Verification items for the finished model (mm, model axes). A direction names the side the tool comes from. Round coordinates to 2 decimals unless told otherwise and drop trailing zeros. Write each loop counter-clockwise with the first axis right and the second up, starting at its lowest first coordinate (ties: lowest second). Pieces come first, ordered by that corner, then holes. Notation, with made-up numbers: (81, 39) - (94, 39) arc R9 ccw to (94, 55) - close; hole circle Ø2 at (61, 17.5). An arc over 180 degrees is marked (long way). Answer as a JSON object with one key per item and string values. Group by question number.
1) Set-up check for faces 1 (the cylindrical face through (-13.753, 5.143, -125.535)), 2 (the flat face through (-72, 10, -123)), 3 (the flat face through (-72, 5, -128)), 4 (the flat face through (-95, 15, -128)): record each of +Z, -Z, +X, -X, +Y, -Y from which the full face is reachable in a straight line by a thin tool's end or side.
2) Mould release check, pull along X, two halves, no side actions. Record for faces 5 (the flat face through (-95, 10, -148)), 6 (the flat face through (-44, 14.9, -120.7)), 7 (the flat face through (-90, 14.9, -170.7)): +X half, -X half, draft (parallel to the pull), parting line (faces both ways), or undercut.
3) Section check D-D (x = -82). Enter the section's corners in (y, z).
4) Section check C-C (z = -16). Enter the section's corners in (x, y).
5) Thickness scan on line 1 (Z direction, x = -81.5, y = 8.75); line 2 (Z direction, x = -67, y = 3.25); line 3 (X direction, y = 8.2, z = -31). Record the ranges inside material, lowest first.
6) Section check B-B (z = -154). Enter the section's corners in (x, y).
7) Section check A-A (x = -5). Enter the section's corners in (y, z).
8) Go/stop test with flat-tipped pins: pin 1 Ø3 at (x, z) = (-27.5, -122.5) entering from +Y; pin 2 Ø11 at (x, y) = (-19.5, 4) entering from -Z; pin 3 Ø11 at (x, y) = (-50.5, 17.5) entering from +Z. Record where each tip stops, or that it passes through.
Autodesk Inventor part; units mm, degrees
ref_plane "YZ Plane" through (0, 0, 0) normal (1, 0, 0) x (0, 1, 0)
ref_plane "XZ Plane" through (0, 0, 0) normal (0, 1, 0) x (-1, 0, 0)
ref_plane "XY Plane" through (0, 0, 0) normal (0, 0, 1) x (1, 0, 0)
sketch "Sketch1" plane through (0, 0, 0) normal (0, 1, 0) x (-1, 0, 0)
  line L0 (0, 0) -> (100, 0)
  line L1 (100, 0) -> (100, -178)
  line L2 (0, -178) -> (0, 0)
  line L3 (90, -10) -> (10, -10)
  line L4 (90, -52) -> (10, -52)
  line L5 (90, -62) -> (10, -62)
  line L6 (90, -52) -> (90, -10)
  line L7 (10, -10) -> (10, -52)
  line L8 (90, -118) -> (10, -118)
  line L9 (90, -168) -> (90, -128)
  line L10 (90, -118) -> (90, -62)
  line L11 (10, -62) -> (10, -118)
  line L12 (10, -128) -> (10, -168)
  line L13 (100, -178) -> (90, -178)
  line L14 (10, -178) -> (0, -178)
  line L15 (90, -168) -> (90, -178)
  line L16 (10, -168) -> (44, -168)
  line L17 (54, -168) -> (54, -178)
  line L18 (54, -178) -> (10, -178)
  line L19 (54, -168) -> (54, -128)
  line L20 (44, -128) -> (44, -168)
  line L21 (90, -128) -> (54, -128)
  line L22 (44, -128) -> (10, -128)
  dimension "thickness" = 10
  dimension "d3" = 10
  dimension "d4" = 10
  dimension "d8" = 10
  dimension "motor" = 42
  dimension "d10" = 10
  dimension "d11" = 10
  dimension "d27" = 10
  dimension "batterywidth" = 56
  dimension "d31" = 80
  dimension "suspensionWidth" = 40
  dimension "d33" = 10
  dimension "d34" = 10
  dimension "d36" = 10
  dimension "d38" = 10
  dimension "d39" = 40
  dimension "d40" = 40
  dimension "d41" = 34
  dimension "d215" = 36
extrude "Extrusion2" add sketch "Sketch1" along normal blind 10
sketch "Sketch2" plane through (0, 10, 0) normal (0, 1, 0) x (1, 0, 0)
  line L0 (-100, 0) -> (-90, 0)
  line L1 (-90, 0) -> (-90, 10)
  line L2 (-90, 10) -> (-100, 10)
  line L3 (-100, 10) -> (-100, 0)
  line L4 (-10, 52) -> (-10, 10)
  line L5 (0, 0) -> (-10, 0)
  line L6 (-10, 0) -> (-10, 10)
  line L7 (-10, 10) -> (0, 10)
  line L8 (0, 10) -> (0, 0)
  line L9 (-100, 178) -> (-100, 0)
  line L10 (-100, 0) -> (0, 0)
  line L11 (-100, 52) -> (-90, 52)
  line L12 (-90, 52) -> (-90, 62)
  line L13 (-90, 62) -> (-100, 62)
  line L14 (-100, 62) -> (-100, 52)
  line L15 (-90, 52) -> (-10, 52)
  line L16 (-10, 52) -> (0, 52)
  line L17 (0, 52) -> (0, 62)
  line L18 (0, 62) -> (-10, 62)
  line L19 (-10, 62) -> (-10, 52)
  line L20 (-90, 10) -> (-90, 52)
  line L21 (-100, 118) -> (-90, 118)
  line L22 (-90, 118) -> (-90, 128)
  line L23 (-90, 128) -> (-100, 128)
  line L24 (-100, 128) -> (-100, 118)
  line L25 (-54, 128) -> (-90, 128)
  line L26 (-54, 118) -> (-44, 118)
  line L27 (-44, 118) -> (-44, 128)
  line L28 (-44, 128) -> (-54, 128)
  line L29 (-54, 128) -> (-54, 118)
  line L30 (-90, 118) -> (-10, 118)
  line L31 (0, 178) -> (-54, 178)
  line L32 (-10, 168) -> (0, 168)
  line L33 (0, 168) -> (0, 178)
  line L34 (0, 178) -> (-10, 178)
  line L35 (-10, 178) -> (-10, 168)
  line L36 (0, 0) -> (0, 178)
  line L37 (-10, 118) -> (0, 118)
  line L38 (0, 118) -> (0, 128)
  line L39 (0, 128) -> (-10, 128)
  line L40 (-10, 128) -> (-10, 118)
  line L41 (-10, 128) -> (-44, 128)
  line L42 (-54, 158) -> (-44, 158)
  line L43 (-44, 158) -> (-44, 168)
  line L44 (-44, 168) -> (-54, 168)
  line L45 (-54, 168) -> (-54, 158)
  line L46 (-44, 168) -> (-10, 168)
  line L47 (-44, 128) -> (-44, 168)
  line L48 (-100, 158) -> (-90, 158)
  line L49 (-90, 158) -> (-90, 168)
  line L50 (-90, 168) -> (-100, 168)
  line L51 (-100, 168) -> (-100, 158)
  line L52 (-90, 128) -> (-90, 178)
  dimension "d34" = 10
  dimension "d44" = 10
  dimension "d45" = 10
  dimension "d47" = 10
  dimension "d50" = 10
  dimension "d51" = 10
  dimension "d52" = 10
  dimension "d53" = 10
  dimension "d58" = 10
  dimension "d64" = 10
  dimension "d65" = 10
  dimension "d148" = 10
  dimension "d149" = 10
  dimension "d150" = 10
  dimension "d151" = 10
extrude "Extrusion3" add sketch "Sketch2" along normal blind 10 contours L3 L2 L1 L0 | L6 L7 L8 L5 | L9 L13 L12 L11 | L19 L18 L17 L16 | L9 L23 L22 L21 | L9 L50 L49 L48 | L29 L28 L27 L26 | L37 L40 L39 L36 | L32 L35 L31 L33 | L42 L45 L44 L43
sketch "Sketch6" plane through (0, 0, 0) normal (0, -1, 0) x (1, 0, 0)
  line L0 (-90, -10) -> (-80, -10)
  line L1 (-80, -10) -> (-80, -52)
  line L2 (-80, -52) -> (-90, -52)
  line L3 (-90, -52) -> (-90, -10)
  line L4 (-90, -52) -> (-90, -10)
  line L5 (-90, -10) -> (-10, -10)
  line L6 (-10, -52) -> (-90, -52)
  line L7 (-20, -10) -> (-10, -10)
  line L8 (-10, -10) -> (-10, -52)
  line L9 (-10, -52) -> (-20, -52)
  line L10 (-20, -52) -> (-20, -10)
  line L11 (-10, -10) -> (-10, -52)
  point P0 (0, 0)
  dimension "motorFixtureHeight" = 60
  dimension "d72" = 10
extrude "Extrusion5" add sketch "Sketch6" against normal blind 10 contours L0 L1 L2 L3 | L5 L8 L6 L10
sketch "Sketch7" plane through (0, 10, 0) normal (0, 1, 0) x (1, 0, 0)
  line L0 (-80, 10) -> (-20, 10)
  line L1 (-20, 10) -> (-20, 52)
  line L2 (-20, 52) -> (-80, 52)
  line L3 (-80, 52) -> (-80, 10)
  line L4 (-80, 10) -> (-80, 52)
  line L5 (-80, 52) -> (-20, 52)
  line L6 (-20, 52) -> (-20, 10)
  line L7 (-20, 10) -> (-80, 10)
  circle A0 centre (-50, 31) radius 18.75
  circle A1 centre (-75, 16) radius 2.1
  circle A2 centre (-25, 31) radius 2.1
  circle A3 centre (-75, 46) radius 2.1
  circle A4 centre (-25, 16) radius 2.1
  circle A5 centre (-25, 46) radius 2.1
  circle A6 centre (-75, 31) radius 2.1
  point P0 (0, 0)
  dimension "d75" = 37.5
  dimension "d77" = 21
  dimension "d78" = 30
  dimension "d79" = 4.2
  dimension "d80" = 4.2
  dimension "d82" = 4.2
  dimension "d83" = 4.2
  dimension "d84" = 4.2
  dimension "d85" = 4.2
  dimension "d86" = 25
  dimension "d87" = 0
  dimension "d88" = 25
  dimension "d89" = 15
  dimension "d90" = 25
  dimension "d91" = 15
  dimension "d92" = 15
  dimension "d93" = 25
  dimension "d94" = 25
  dimension "d95" = 0
  dimension "d96" = 25
  dimension "d97" = 15
extrude "Extrusion6" add sketch "Sketch7" against normal blind 6
hole "Hole2" at (0, 15, -173) direction (-1, 0, 0) diameter 4.3 end through all
hole "Hole3" at (0, 15, -123) direction (-1, 0, 0) diameter 4.3 end through all
hole "Hole4" at (0, 15, -57) direction (-1, 0, 0) diameter 4.3 end through all
hole "Hole5" at (0, 15, -5) direction (-1, 0, 0) diameter 4.3 end through all
sketch "Sketch8" plane through (-100, 0, -178) normal (-1, 0, 0) x (0, 0, 1)
  line L0 (116, 10) -> (60, 10)
  line L1 (60, 10) -> (60, 7)
  line L2 (60, 7) -> (116, 7)
  line L3 (116, 7) -> (116, 10)
  line L4 (116, 10) -> (60, 7) construction
  line L5 (60, 10) -> (116, 7) construction
  line L6 (60, 10) -> (116, 10)
  line L7 (60, 10) -> (60, 20)
  line L8 (116, 10) -> (116, 20)
  point P0 (178, 0)
  point P1 (88, 8.5)
  dimension "d145" = 3
extrude "Extrusion7" cut sketch "Sketch8" against normal up to surface (100 mm away)
hole "Hole6" at (-95, 15, -168) direction (0, 0, 1) diameter 4.3 depth 10 tip angle 118
hole "Hole7" at (-49, 15, -168) direction (0, 0, 1) diameter 4.3 depth 10 tip angle 118
sketch "Sketch10" plane through (0, 0, 0) normal (0, -1, 0) x (1, 0, 0)
  line L0 (-90, -168) -> (-54, -168)
  line L1 (-54, -168) -> (-54, -178)
  line L2 (-54, -178) -> (-90, -178)
  line L3 (-90, -178) -> (-90, -168)
  line L4 (-54, -128) -> (-54, -178)
  line L5 (-90, -178) -> (-90, -128)
  line L6 (-10, -168) -> (-44, -168)
  line L7 (-54, -178) -> (0, -178)
  point P0 (0, 0)
extrude "Extrusion9" add sketch "Sketch10" against normal blind 10
sketch "Sketch11" plane through (0, 0, 0) normal (0, -1, 0) x (1, 0, 0)
  line L0 (-44, -168) -> (-10, -168)
  line L1 (-10, -168) -> (-10, -178)
  line L2 (-10, -178) -> (-44, -178)
  line L3 (-44, -178) -> (-44, -168)
  line L4 (-10, -168) -> (-44, -168)
  line L5 (-100, -178) -> (0, -178)
  line L6 (-44, -168) -> (-44, -128)
  line L7 (-10, -128) -> (-10, -168)
  point P0 (0, 0)
extrude "Extrusion10" cut sketch "Sketch11" against normal blind 10
sketch "Sketch12" plane through (-10, 0, -128) normal (0, 0, -1) x (-1, 0, 0)
  circle A0 centre (27, 5) radius 3.25
  circle A1 centre (7, 5) radius 3.25
  line L0 (34, 0) -> (0, 0)
  line L1 (34, 10) -> (34, 0)
  line L2 (0, 0) -> (0, 20)
  point P0 (-10, 0)
  dimension "d182" = 6.5
  dimension "d183" = 6.5
  dimension "d184" = 5
  dimension "d185" = 7
  dimension "d186" = 7
  dimension "d187" = 5
extrude "Extrusion11" cut sketch "Sketch12" against normal blind 5
sketch "Sketch13" plane through (0, 20, 0) normal (0, 1, 0) x (1, 0, 0)
  line L0 (-100, 158) -> (-90, 158)
  line L1 (-90, 158) -> (-90, 168)
  line L2 (-90, 168) -> (-100, 168)
  line L3 (-100, 168) -> (-100, 158)
  line L4 (-90, 168) -> (-100, 168)
  line L5 (-90, 158) -> (-90, 168)
  line L6 (-100, 168) -> (-100, 158)
  line L7 (-100, 158) -> (-90, 158)
  line L8 (-10, 168) -> (0, 168)
  line L9 (0, 168) -> (0, 178)
  line L10 (0, 178) -> (-10, 178)
  line L11 (-10, 178) -> (-10, 168)
  line L12 (-10, 178) -> (-10, 168)
  line L13 (0, 178) -> (-10, 178)
  line L14 (0, 168) -> (0, 178)
  line L15 (-10, 168) -> (0, 168)
  point P0 (0, 0)
extrude "Extrusion12" cut sketch "Sketch13" against normal blind 10
sketch "Sketch14" plane through (0, 10, 0) normal (0, 1, 0) x (1, 0, 0)
  line L0 (-10, 158) -> (0, 158)
  line L1 (0, 158) -> (0, 168)
  line L2 (0, 168) -> (-10, 168)
  line L3 (-10, 168) -> (-10, 158)
  line L4 (-10, 178) -> (0, 178)
  line L5 (-10, 128) -> (-10, 178)
  line L6 (-90, 168) -> (-54, 168)
  line L7 (0, 128) -> (0, 178)
  line L8 (-100, 168) -> (-90, 168)
  line L9 (-90, 168) -> (-90, 178)
  line L10 (-90, 178) -> (-100, 178)
  line L11 (-100, 178) -> (-100, 168)
  line L12 (-44, 178) -> (-100, 178)
  line L13 (-100, 178) -> (-100, 128)
  line L14 (-90, 128) -> (-90, 168)
  line L15 (-54, 158) -> (-44, 158)
  point P0 (0, 0)
  dimension "d192" = 10
  dimension "d193" = 10
  dimension "d194" = 10
extrude "Extrusion13" add sketch "Sketch14" along normal blind 10 contours L3 L2 L1 L0 | L11 L10 L9 L8
hole "Hole8" at (-5, 15, -168) direction (0, 0, 1) diameter 4.3 depth 10 tip angle 118
hole "Hole9" at (-100, 15, -173) direction (1, 0, 0) diameter 4.3 depth 10 tip angle 118
equation "\"d3\" = thickness"
equation "\"d4\" = thickness"
equation "\"d8\" = thickness"
equation "\"d10\" = thickness"
equation "\"d11\" = thickness"
equation "\"d27\" = thickness"
equation "\"d33\" = thickness"
equation "\"d34\" = thickness"
equation "\"d36\" = thickness"
equation "\"d38\" = thickness"
equation "\"d39\" = suspensionWidth"
equation "\"d40\" = suspensionWidth"
equation "\"d42\" = thickness"
equation "\"d44\" = thickness"
equation "\"d50\" = thickness"
equation "\"d51\" = thickness"
equation "\"d52\" = thickness"
equation "\"d53\" = thickness"
equation "\"d58\" = thickness"
equation "\"d64\" = thickness"
equation "\"d65\" = thickness"
equation "\"d148\" = thickness"
equation "\"d149\" = thickness"
equation "\"d150\" = thickness"
equation "\"d151\" = thickness"
equation "\"d66\" = thickness"
equation "\"d73\" = thickness"
equation "\"d77\" = 0.5 * motor"
equation "\"d159\" = thickness"
equation "\"d168\" = thickness"
properties part number "sideFrame2" material "ABS Plastic"
Returned:
{
 "1": {"face 1": "-Z", "face 2": "+Z, -Z, +Y", "face 3": "+Y, -Y", "face 4": "+X, -X, +Y"},
 "2": {"face 5": "draft", "face 6": "undercut", "face 7": "+X half"},
 "3": {"outline": "(0, -178) - (10, -178) - (10, -168) - (0, -168) - close; (0, -128) - (10, -128) - (10, -118) - (0, -118) - close; (0, -62) - (10, -62) - (10, 0) - (0, 0) - close"},
 "4": {"outline": "(-100, 0) - (-80, 0) - (-80, 4) - (-77.1, 4) - (-77.1, 10) - (-100, 10) - close; (-72.9, 4) - (-61.25, 4) - (-61.25, 10) - (-72.9, 10) - close; (-38.75, 4) - (-27.1, 4) - (-27.1, 10) - (-38.75, 10) - close; (-22.9, 4) - (-20, 4) - (-20, 0) - (0, 0) - (0, 10) - (-22.9, 10) - close"},
 "5": {"line 1": "-178 to -168, -128 to -118, -62 to 0", "line 2": "-178 to -168, -128 to -118, -62 to -52, -10 to 0", "line 3": "-100 to -77.1, -72.9 to -68.75, -31.25 to -27.1, -22.9 to 0"},
 "6": {"outline": "(-100, 0) - (-90, 0) - (-90, 10) - (-100, 10) - close; (-54, 0) - (-44, 0) - (-44, 10) - (-54, 10) - close; (-10, 0) - (0, 0) - (0, 10) - (-10, 10) - close"},
 "7": {"outline": "(0, -178) - (10, -178) - (10, -168) - (12.85, -168) - (12.85, -158) - (10, -158) - (10, -128) - (20, -128) - (20, -118) - (7, -118) - (7, -62) - (20, -62) - (20, -52) - (10, -52) - (10, -10) - (20, -10) - (20, 0) - (0, 0) - close; (17.15, -168) - (20, -168) - (20, -158) - (17.15, -158) - close; hole circle Ø4.3 at (15, -123); hole circle Ø4.3 at (15, -57); hole circle Ø4.3 at (15, -5)"},
 "8": {"pin 1": "y = 10", "pin 2": "z = -128", "pin 3": "z = -118"}
}
